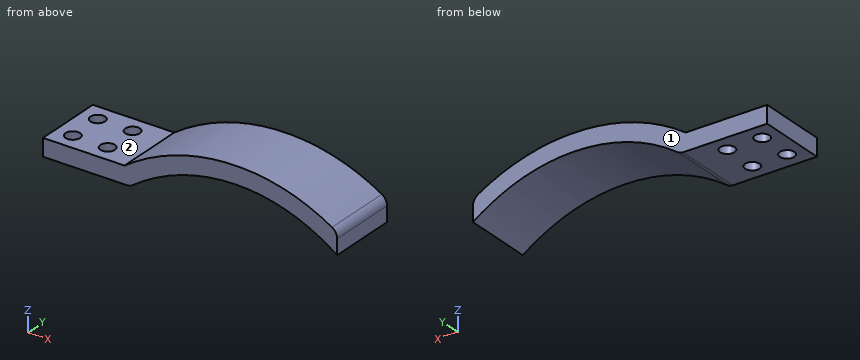
Autodesk Inventor part; units mm, degrees
ref_plane "YZ Plane" through (0, 0, 0) normal (1, 0, 0) x (0, 1, 0)
ref_plane "XZ Plane" through (0, 0, 0) normal (0, 1, 0) x (-1, 0, 0)
ref_plane "XY Plane" through (0, 0, 0) normal (0, 0, 1) x (1, 0, 0)
sketch "Sketch1" plane through (0, 0, 0) normal (0, 1, 0) x (-1, 0, 0)
  line L0 (0, 0) -> (-25, 0)
  spline S0 degree 4 poles (-25, 0) (-32.0397, 5.1858) (-46.8322, 11.6047) (-63.1678, 11.6047) (-77.9603, 5.1858) (-85, 0) knots 0 0 0 0 0 0.5 1 1 1 1 1
  line L1 (-48.6479, 10) -> (-61.3521, 10) construction
  arc A0 (-49.9441, 9.7453) -> (-60.0559, 9.7453) centre (-55, -40.3178) ccw construction
  line L2 (-55, -16.2069) -> (-55, 34.9248) construction
  line L3 (-70, -22.2053) -> (-70, 28.9302) construction
  circle A1 centre (-55, -40) radius 50 construction
  line L4 (-23.3959, 5) -> (0, 5)
  line L5 (-84.476, 6.4124) -> (-84.476, 0)
  line L6 (-84.476, 0) -> (-85, 0)
  line L7 (0, 5) -> (0, 0)
  spline S1 degree 5 poles (-84.476, 6.4124) (-81.1502, 8.5173) (-77.647, 10.3417) (-73.9852, 11.8448) (-65.816, 14.3543) (-57.3038, 15.2371) (-52.6962, 15.2371) (-43.673, 14.3013) (-35.0354, 11.5377) (-30.933, 9.7391) (-27.0473, 7.5377) (-23.3959, 4.9999) knots 0 0 0 0 0 0 0.303739 0.303739 0.303739 0.656836 0.656836 0.656836 1 1 1 1 1 1
  point P0 (-40, 7.697)
  point P1 (-55, 10)
  point P2 (-70, 7.697)
  point P3 (-84.476, 0.3814)
  dimension "d5" = 5
  dimension "d0" = 60
  dimension "d1" = 25
  dimension "d2" = 100
extrude "Extrusion1" add sketch "Sketch1" along normal blind 20 contours L0 S0 L5 S1 L4 L7
sketch "Sketch2" plane through (25, 0, 0) normal (0, 0, -1) x (-1, 0, 0)
  circle A0 centre (10, 15) radius 2.1
  line L0 (0, 20) -> (25, 20)
  line L1 (0, 0) -> (25, 0)
  line L2 (25, 0) -> (25, 20)
  line L3 (0, 20) -> (25, 20)
  line L4 (0, 0) -> (0, 20)
  circle A1 centre (20, 15) radius 2.1
  circle A2 centre (10, 5) radius 2.1
  circle A3 centre (20, 5) radius 2.1
  dimension "d8" = 4.2
  dimension "d11" = 10
  dimension "d14" = 10
  dimension "d17" = 10
  dimension "d18" = 5
extrude "Extrusion2" cut sketch "Sketch2" against normal up to surface (5 mm away) contours A0 | A1 | A2 | A3
fillet "Fillet1" radius 3 1 edges at (84.476, 10, 6.4124)
fillet "Fillet2" radius 2.5 1 edges at (25, 10, 0)
properties part number "Gripper_Concave_Finger"
The model under review builds one solid part; all positions refer to its coordinate system, in mm. Face numbers are marked on the shaded views. A direction names the side the tool comes from. Round coordinates to 2 decimals unless told otherwise and drop trailing zeros. Loops run counter-clockwise (first coordinate to the right, second up) from the corner with the lowest first, then second, coordinate; pieces in that order, holes last. Notation, with made-up numbers: (4, -26) -> (29, -26) arc R31 ccw to (29, 8) -> close; hole circle Ø8 at (-2, -21.75). An arc over 180 degrees is marked (long way). Answer as a JSON object with one key per item and string values. Group by question number.
1) For the marked faces 1 and 2, list the 3-axis set-ups (+Z, -Z, +X, -X, +Y, -Y) from which the entire face can be reached by the end or side of a thin tool; tool diameter is ignored.
2) For line 1 (Y direction, x = 5, z = 1.65); line 2 (Y direction, x = 6, z = 4); line 3 (Z direction, x = 55, y = 11.75), list the stretches that pass through material, from the lowest coordinate up. Write a range as [from, to].
3) We need section A-A on x = 5. Write out the cut boundary in (y, z), then the cut area to 3 significant figures.
4) We need section B-B on y = 15. Give the number of separate pieces and of enclosed holes in the cut face, then the cut area to 3 significant figures.
5) For pin 1 Ø2 at (y, z) = (12, 10) entering from -X; pin 2 Ø2 at (x, y) = (32.5, 14) entering from +Z; pin 3 Ø6 at (x, y) = (10, 13.5) entering from +Z, all flat-tipped, find the tip position at first contact; note any pin that passes through.
Result set:
{
 "1": {"face 1": "+Z, -Z, +X, -X, +Y", "face 2": "+Z, -X, +Y, -Y"},
 "2": {"line 1": "[0, 2.9], [7.1, 12.9], [17.1, 20]", "line 2": "[0, 3.15], [6.85, 13.15], [16.85, 20]", "line 3": "[10, 15]"},
 "3": {"outline": "(0, 0) -> (2.9, 0) -> (2.9, 5) -> (0, 5) -> close; (7.1, 0) -> (12.9, 0) -> (12.9, 5) -> (7.1, 5) -> close; (17.1, 0) -> (20, 0) -> (20, 5) -> (17.1, 5) -> close", "area": "58.0 mm²"},
 "4": {"separate pieces": "3", "enclosed holes": "0", "area": "400 mm²"},
 "5": {"pin 1": "x = 30.06", "pin 2": "z = 10.61", "pin 3": "z = 5"}
}
